from build123d import *

# Parameters (mm, degrees)
SKETCH003_W  = 44
SKETCH003_H  = 48
PAD002_DEPTH = 61
SKETCH004_W  = 44
SKETCH004_H  = 48
PAD003_DEPTH = 3
SKETCH005_R  = 1.25
POCKET_DEPTH = 30


with BuildPart() as part:
    # Sketch003 (on Face1 of Binder004) → Pad002 (new body)
    with BuildSketch(Plane.XZ.offset(-30.5)):
        with Locations((0, -2)):
            Rectangle(SKETCH003_W, SKETCH003_H)
        with BuildLine():
            Line((-16.5, -23), (16.5, -23))
            ThreePointArc((19, -20.5), (17.232233, -21.232233), (16.5, -23))
            Line((19, -20.5), (19, 16.499999))
            ThreePointArc((16.5, 18.999999), (17.232233, 17.232232), (19, 16.499999))
            Line((16.5, 18.999999), (-16.5, 18.999999))
            ThreePointArc((-19, 16.5), (-17.232233, 17.232233), (-16.5, 18.999999))
            Line((-19, 16.5), (-19, -20.5))
            ThreePointArc((-16.5, -23), (-17.232233, -21.232233), (-19, -20.5))
        make_face(mode=Mode.SUBTRACT)
    extrude(amount=PAD002_DEPTH)

    # Sketch004 (on Face14 of Pad002) → Pad003 (join)
    with BuildSketch(Plane.XZ.offset(30.5)):
        with Locations((0, -2)):
            Rectangle(SKETCH004_W, SKETCH004_H)
    extrude(amount=PAD003_DEPTH)

    # Sketch005 (on Face1 of Pad003) → Pocket (cut)
    with BuildSketch(Plane(origin=(0, 30.5, 0), x_dir=(-1, 0, 0), z_dir=(0, 1, 0))):
        with Locations((-19.462404, 19.260412)):
            Circle(SKETCH005_R)
        with Locations((19.271234, 19.432414)):
            Circle(SKETCH005_R)
        with Locations((19.271234, -23.428404)):
            Circle(SKETCH005_R)
        with Locations((-19.428404, -23.271234)):
            Circle(SKETCH005_R)
    extrude(amount=-POCKET_DEPTH, mode=Mode.SUBTRACT)


solid = part.part
Verification items for the finished model (mm, model axes). A direction names the side the tool comes from. Round coordinates to 2 decimals unless told otherwise and drop trailing zeros. Loops run counter-clockwise (first coordinate to the right, second up) from the corner with the lowest first, then second, coordinate; pieces in that order, holes last. Notation, with made-up numbers: (7.5, -37.5) - (62.5, -37.5) arc R10 cw to (62.5, -21.5) - close; hole circle Ø11 at (84, -8.75). An arc over 180 degrees is marked (long way). Write item = value, one per line.
Q1. Mould release check, pull along Z, two halves, no side actions. Record for faces 3 (the flat face through (0, -1, 22)), 4 (the cylindrical face through (-20.464, 15.71, 19.808)), 5 (the flat face through (-20, 30.5, 0)): +Z half, -Z half, draft (parallel to the pull), parting line (faces both ways), or undercut.
Here are the results:
face_3 = +Z half
face_4 = undercut
face_5 = draft
Q2. Sectioned sample at C-C on x = 0. Record the boundary of the cut face in (y, z).
Here are the results:
outline = (-33.5, -26) - (30.5, -26) - (30.5, -23) - (-30.5, -23) - (-30.5, 19) - (30.5, 19) - (30.5, 22) - (-33.5, 22) - close
Q3. Sectioned sample at D-D on y = 21. Record the boundary of the cut face in (x, z), plus the area to 3 significant figures.
Here are the results:
outline = (-22, -26) - (22, -26) - (22, 22) - (-22, 22) - close; hole circle Ø2.5 at (-19.27, -23.43); hole circle Ø2.5 at (-19.27, 19.43); hole (-19, -20.5) arc R2.5 cw to (-16.5, -23) - (16.5, -23) arc R2.5 cw to (19, -20.5) - (19, 16.5) arc R2.5 cw to (16.5, 19) - (-16.5, 19) arc R2.5 cw to (-19, 16.5) - close; hole circle Ø2.5 at (19.43, -23.27); hole circle Ø2.5 at (19.46, 19.26)
area = 516 mm^2
Q4. Sectioned sample at B-B on z = -13.5. Record the boundary of the cut face in (x, y), plus the area to 3 significant figures.
Here are the results:
outline = (-22, -33.5) - (22, -33.5) - (22, 30.5) - (19, 30.5) - (19, -30.5) - (-19, -30.5) - (-19, 30.5) - (-22, 30.5) - close
area = 498 mm^2
Q5. Material ranges on L1, parallel to Z at x = 15.5, y = -27.5; L2, parallel to X at y = 20.5, z = -5; L3, parallel to Y at x = -3, z = -17, recorded low to high.
Here are the results:
L1 = -26 to -23, 19 to 22
L2 = -22 to -19, 19 to 22
L3 = -33.5 to -30.5
Q6. Sectioned sample at A-A on y = -27. Record the boundary of the cut face in (x, z).
Here are the results:
outline = (-22, -26) - (22, -26) - (22, 22) - (-22, 22) - close; hole (-19, -20.5) arc R2.5 cw to (-16.5, -23) - (16.5, -23) arc R2.5 cw to (19, -20.5) - (19, 16.5) arc R2.5 cw to (16.5, 19) - (-16.5, 19) arc R2.5 cw to (-19, 16.5) - close
Q7. Depth check by flat-ended pin: pin 1 (1.5 mm diameter, centred on x = 6, z = 0.5, fed in from +Y); pin 2 (3 mm diameter, centred on x = 19, z = -23, fed in from +Y). Enter the tip coordinate at first touch or a pass-through.
Here are the results:
pin_1 = -30.5
pin_2 = 30.5
Q8. Tool access check on faces 1 (the flat face through (0, 0, 19)), 2 (the flat face through (22, -1, -2)). Record the directions out of +Z, -Z, +X, -X, +Y, -Y that give a thin tool (end or side, any length) a straight path to the whole face; none if there is none.
Here are the results:
face_1 = +Y
face_2 = +Z, -Z, +X, +Y, -Y
